Source: CAD feature listing. Evaluate the final solid. Frame: model axes, mm. Face numbers are marked on the shaded views. A direction names the side the tool comes from. Round coordinates to 2 decimals unless told otherwise and drop trailing zeros. Write each loop counter-clockwise with the first axis right and the second up, starting at its lowest first coordinate (ties: lowest second). Pieces come first, ordered by that corner, then holes. Notation, with made-up numbers: M -21.5,25.25 L 29.5,25.25 A19 cw 29.5,56.25 Z; hole C 46.5,7 d5. An arc over 180 degrees is marked long. Answer in a Markdown table with one row per item. Add a question column.
Item 1: Cut plane B-B on z = 0. Return loops of the section in (x, y), and give its area (3 significant figures).
Item 2: Cut plane D-D on x = -14. Return loops of the section in (y, z), and give its area (3 significant figures).
Item 3: Set-up query: the marked faces 1, 2, 3, 4 and 5. Return all of +Z, -Z, +X, -X, +Y, -Y with unobstructed straight access to the full face (end or side cutting, diameter ignored); none if empty.
Item 4: Cut plane C-C on y = 1.75. Return loops of the section in (x, z), and give its area (3 significant figures).
Item 5: Material intervals for probe 1 along X at (y, z) = (3.75, 0); probe 2 along Z at (x, y) = (0, 3); probe 3 along Y at (x, z) = (16, -8), sorted ascending.
Item 6: Contact query for flat-ended pins moving along their axis: pin 1 (1 mm diameter, centred on x = -13.5, y = 3.5, fed in from -Z); pin 2 (10 mm diameter, centred on x = -23.5, z = -45, fed in from -Y); pin 3 (5 mm diameter, centred on y = 3, z = -65, fed in from -X); pin 4 (1.5 mm diameter, centred on y = 8, z = -46, fed in from +X). Output: stop coordinate, or through.
Item 7: Cut plane A-A on x = 0. Return loops of the section in (y, z), and give its area (3 significant figures).
Item 8: Mould query, pull axis X, two halves, no side actions, for the marked faces 6, 7, 8 and 9. Classes: released by +X, released by -X, zero draft, split by the parting line, or undercut.
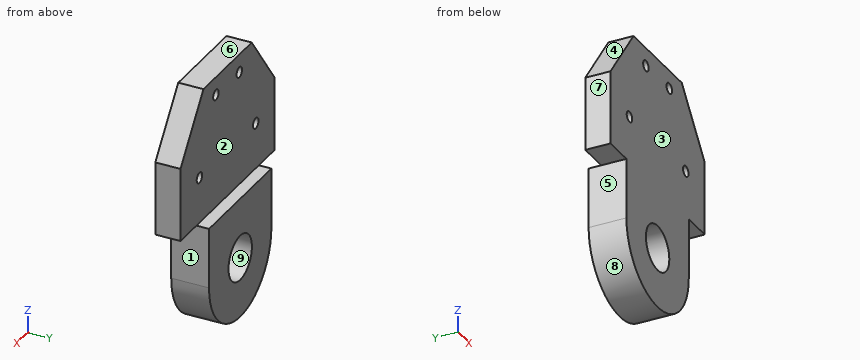
from build123d import *

# Parameters (mm, degrees)
SKETCH1_R           = 1.75
BOSS_EXTRUDE1_DEPTH = 8.333333333
SKETCH2_R           = 7.5
BOSS_EXTRUDE2_DEPTH = 12.5


with BuildPart() as part:
    # Sketch1 → Boss-Extrude1 (new body)
    with BuildSketch(Plane(origin=(0, 0, 0), x_dir=(1, 0, 0), z_dir=(0, 1, 0))):
        Polygon((-30.225021847, 13.45402847), (-15.473485445, -6.035190955), (15.473485445, -6.035190955), (30.225021847, 13.45402847), (30.225021847, 37.907694676), (18.065456544, 37.907694676), (-18.065456544, 37.907694676), (-30.225021847, 37.907694676), align=None)
        with Locations((-18.065456544, 22.657694676)):
            Circle(SKETCH1_R, mode=Mode.SUBTRACT)
        with Locations((18.065456544, 22.657694676)):
            Circle(SKETCH1_R, mode=Mode.SUBTRACT)
        with Locations((7.5, 0)):
            Circle(SKETCH1_R, mode=Mode.SUBTRACT)
        with Locations((-7.5, 0)):
            Circle(SKETCH1_R, mode=Mode.SUBTRACT)
    extrude(amount=BOSS_EXTRUDE1_DEPTH)

    # Sketch2 → Boss-Extrude2 (add)
    with BuildSketch(Plane(origin=(0, 0, 0), x_dir=(1, 0, 0), z_dir=(0, 1, 0))):
        with BuildLine():
            Line((-20, 57.907694676), (-20, 37.907694676))
            Line((-20, 37.907694676), (20, 37.907694676))
            Line((20, 37.907694676), (20, 57.907694676))
            ThreePointArc((20, 57.907694676), (0, 77.907694676), (-20, 57.907694676))
        make_face()
        with Locations((0, 57.907694676)):
            Circle(SKETCH2_R, mode=Mode.SUBTRACT)
    extrude(amount=BOSS_EXTRUDE2_DEPTH)


solid = part.part
Results below:
| question | item | result |
|---|---|---|
| 1 | outline | M -20.04,0 L -9.25,0 L -9.25,8.33 L -20.04,8.33 Z; M -5.75,0 L 5.75,0 L 5.75,8.33 L -5.75,8.33 Z; M 9.25,0 L 20.04,0 L 20.04,8.33 L 9.25,8.33 Z |
| 1 | area | 276 mm2 |
| 2 | outline | M 0,-72.19 L 12.5,-72.19 L 12.5,-37.91 L 8.33,-37.91 L 8.33,6.04 L 0,6.04 Z |
| 2 | area | 795 mm2 |
| 3 | face 1 | -Z, +X, +Y, -Y |
| 3 | face 2 | +Z, +X, -X, +Y |
| 3 | face 3 | +Z, -Z, +X, -X, -Y |
| 3 | face 4 | +Z, -X, +Y, -Y |
| 3 | face 5 | -Z, -X, +Y, -Y |
| 4 | outline | M -30.23,-37.91 L -20,-37.91 L -20,-57.91 A20 ccw 20,-57.91 L 20,-37.91 L 30.23,-37.91 L 30.23,-13.45 L 15.47,6.04 L -15.47,6.04 L -30.23,-13.45 Z; hole C -18.07,-22.66 d3.5; hole C -7.5,0 d3.5; hole C 0,-57.91 d15; hole C 7.5,0 d3.5; hole C 18.07,-22.66 d3.5 |
| 4 | area | 3,580 mm2 |
| 5 | probe 1 | -20.04 to -9.25, -5.75 to 5.75, 9.25 to 20.04 |
| 5 | probe 2 | -77.91 to -65.41, -50.41 to 6.04 |
| 5 | probe 3 | 0 to 8.33 |
| 6 | pin 1 | z = -73.11 |
| 6 | pin 2 | y = 0 |
| 6 | pin 3 | x = -19.47 |
| 6 | pin 4 | x = 20 |
| 7 | outline | M 0,-77.91 L 12.5,-77.91 L 12.5,-65.41 L 0,-65.41 Z; M 0,-50.41 L 12.5,-50.41 L 12.5,-37.91 L 8.33,-37.91 L 8.33,6.04 L 0,6.04 Z |
| 7 | area | 679 mm2 |
| 8 | face 6 | zero draft |
| 8 | face 7 | released by -X |
| 8 | face 8 | split by the parting line |
| 8 | face 9 | undercut |
